```python
from build123d import *

# Parameters (mm, degrees)
SKETCH2_R           = 50.8
BOSS_EXTRUDE1_DEPTH = 9.525
SKETCH3_R           = 2.667
CUT_EXTRUDE1_DEPTH  = 10.525
SKETCH4_W           = 6.477
SKETCH4_H           = 6.477
CUT_EXTRUDE2_DEPTH  = 10.525


with BuildPart() as part:
    # Sketch2 → Boss-Extrude1 (new body)
    with BuildSketch(Plane(origin=(0, 0, 0), x_dir=(1, 0, 0), z_dir=(0, 1, 0))):
        Circle(SKETCH2_R)
    extrude(amount=BOSS_EXTRUDE1_DEPTH)

    # Sketch3 → Cut-Extrude1 (cut, through all)
    with BuildSketch(Plane(origin=(0, 9.525, 0), x_dir=(1, 0, 0), z_dir=(0, 1, 0))):
        with Locations((0, -40.64)):
            Circle(SKETCH3_R)
        with Locations((-40.64, 0)):
            Circle(SKETCH3_R)
        with Locations((0, 40.64)):
            Circle(SKETCH3_R)
        with Locations((40.64, 0)):
            Circle(SKETCH3_R)
    extrude(amount=-CUT_EXTRUDE1_DEPTH, mode=Mode.SUBTRACT)

    # Sketch4 → Cut-Extrude2 (cut, through all)
    with BuildSketch(Plane(origin=(0, 9.525, 0), x_dir=(1, 0, 0), z_dir=(0, 1, 0))):
        Rectangle(SKETCH4_W, SKETCH4_H)
    extrude(amount=-CUT_EXTRUDE2_DEPTH, mode=Mode.SUBTRACT)


solid = part.part
```
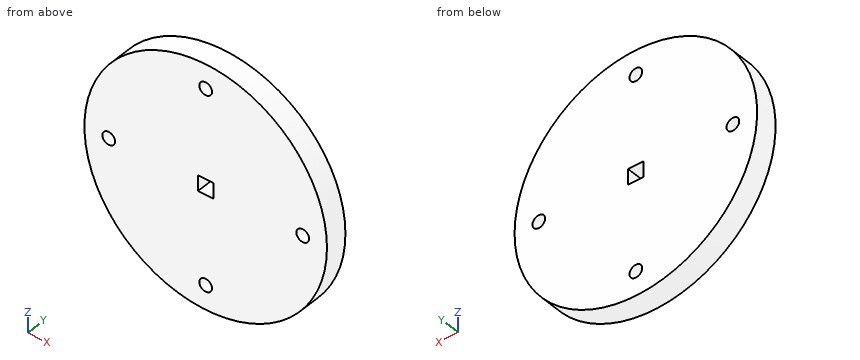
Input: part model. Units: mm. Frame: model coordinates. Coordinates: 2 decimals unless noted, no trailing zeros. Write each loop counter-clockwise with the first axis right and the second up, starting at its lowest first coordinate (ties: lowest second). Pieces come first, ordered by that corner, then holes. Notation, with made-up numbers: (62.5, 3.5) -> (120.5, 3.5) arc R23 cw to (120.5, 11.5) -> close; hole circle Ø2 at (36, 48.25). An arc over 180 degrees is marked (long way). Write each question's results on one line, items separated by ' | '.
Item 1: Section query A-A on z = -40.64. Return loops of the section in (x, y) (3 decimals), plus the area to 3 significant figures.
Conclusion:
outline: (-30.48, 0) -> (-2.667, 0) -> (-2.667, 9.525) -> (-30.48, 9.525) -> close; (2.667, 0) -> (30.48, 0) -> (30.48, 9.525) -> (2.667, 9.525) -> close | area: 530 mm^2
Item 2: Pin query (flat end, axial travel): pin 1 Ø5 at (y, z) = (8, 37.5) entering from -X; pin 2 Ø1.9 at (x, y) = (-1.5, 5) entering from +Z; pin 3 Ø5 at (x, y) = (1.5, 2.5) entering from -Z. Return the tip coordinate at first contact, or that it passes through.
Conclusion:
pin 1: stops at x = -36.82 | pin 2: stops at z = 50.8 | pin 3: stops at z = -50.8
Item 3: Section query D-D on x = 0. Return loops of the section in (y, z) (1 decimal).
Conclusion:
outline: (0, -50.8) -> (9.5, -50.8) -> (9.5, -43.3) -> (0, -43.3) -> close; (0, -38) -> (9.5, -38) -> (9.5, -3.2) -> (0, -3.2) -> close; (0, 3.2) -> (9.5, 3.2) -> (9.5, 38) -> (0, 38) -> close; (0, 43.3) -> (9.5, 43.3) -> (9.5, 50.8) -> (0, 50.8) -> close
Item 4: Material intervals for probe 1 along X at (y, z) = (3, 0); probe 2 along X at (y, z) = (8.5, 2), sorted ascending.
Conclusion:
probe 1: x = -50.8 to -43.31, -37.97 to -3.24, 3.24 to 37.97, 43.31 to 50.8 | probe 2: x = -50.76 to -42.4, -38.88 to -3.24, 3.24 to 38.88, 42.4 to 50.76
Item 5: Section query B-B on x = -40.64. Return loops of the section in (y, z) (3 decimals), plus the area to 3 significant figures.
Conclusion:
outline: (0, -30.48) -> (9.525, -30.48) -> (9.525, -2.667) -> (0, -2.667) -> close; (0, 2.667) -> (9.525, 2.667) -> (9.525, 30.48) -> (0, 30.48) -> close | area: 530 mm^2
Item 6: Section query C-C on y = 4.75. Return loops of the section in (x, z), plus the area to 3 significant figures.
Conclusion:
outline: circle Ø101.6 at (0, 0); hole circle Ø5.33 at (-40.64, 0); hole (-3.24, -3.24) -> (3.24, -3.24) -> (3.24, 3.24) -> (-3.24, 3.24) -> close; hole circle Ø5.33 at (0, -40.64); hole circle Ø5.33 at (0, 40.64); hole circle Ø5.33 at (40.64, 0) | area: 7,980 mm^2
